The listing builds one solid part. Answer for the finished solid, in the listing's coordinates (mm). Face numbers are marked on the shaded views. A direction names the side the tool comes from. Give positions to 0.01 mm unless a question says otherwise; leave off trailing zeros. Write each loop counter-clockwise with the first axis right and the second up, starting at its lowest first coordinate (ties: lowest second). Pieces come first, ordered by that corner, then holes. Notation, with made-up numbers: (-5.75, 79.25) - (40.25, 79.25) arc R18 ccw to (40.25, 109.25) - close; hole circle Ø9 at (-23.75, 58). An arc over 180 degrees is marked (long way). Use a Markdown table: item, result. Add a question column.
from build123d import *

# Parameters (mm, degrees)
SKETCH1_R           = 1.75
SKETCH1_R_2         = 5.75
BOSS_EXTRUDE3_DEPTH = 10
FILLET1_R           = 8
SKETCH6_R           = 3.75
CUT_EXTRUDE2_DEPTH  = 3
FILLET2_R           = 8
FILLET3_R           = 3
SKETCH8_R           = 1.85
CUT_EXTRUDE3_DEPTH  = 69.282336686
SKETCH9_R           = 3.75
CUT_EXTRUDE4_DEPTH  = 4


with BuildPart() as part:
    # Sketch1 → Boss-Extrude3 (new body)
    with BuildSketch(Plane(origin=(20, 0, 0), x_dir=(0, 0, -1), z_dir=(1, 0, 0))):
        with BuildLine():
            Line((-17.699617141, 42.082180663), (-39.499785546, 42.082180663))
            Line((-39.499785546, 42.082180663), (-39.499785546, 32.582180663))
            Line((-39.499785546, 32.582180663), (-18.499785546, 32.582180663))
            Line((-18.499785546, 32.582180663), (-18.499785546, 9))
            Line((-18.499785546, 9), (-41.626388373, 9))
            ThreePointArc((-41.626388373, 9), (-51.838324672, 8.238612788), (-46.499785546, -0.5))
            Line((-46.499785546, -0.5), (-9.499785546, -0.5))
            Line((-9.499785546, -0.5), (-9.499785546, -9.5))
            Line((-9.499785546, -9.5), (9.500214454, -9.5))
            Line((9.500214454, -9.5), (9.500214454, 31.5))
            Line((9.500214454, 31.5), (-9.499785546, 31.5))
            Line((-9.499785546, 31.5), (-9.499785546, 36.5))
            ThreePointArc((-9.499785546, 36.5), (-12.123322128, 41.459787776), (-17.699617141, 42.082180663))
        make_face()
        with Locations((-15.499785546, 36.5)):
            Circle(SKETCH1_R, mode=Mode.SUBTRACT)
        with Locations((0.000214454, 22)):
            Circle(SKETCH1_R_2, mode=Mode.SUBTRACT)
        with Locations((0.000214454, 0)):
            Circle(SKETCH1_R_2, mode=Mode.SUBTRACT)
        with Locations((-15.499785546, 5.5)):
            Circle(SKETCH1_R, mode=Mode.SUBTRACT)
        with Locations((-46.499785546, 5.5)):
            Circle(SKETCH1_R, mode=Mode.SUBTRACT)
    extrude(amount=BOSS_EXTRUDE3_DEPTH)

    # Fillet1
    fillet1_edges = [part.edges().sort_by_distance(p)[0] for p in [
        (25, -9.5, 9.499785546),
        (25, -9.5, -9.500214454),
        (25, 31.5, -9.500214454),
        (25, 9, 18.499785546),
        (25, 31.5, 9.499785546),
        (25, 32.582180663, 18.499785546),
    ]]
    fillet(fillet1_edges, radius=FILLET1_R)

    # Sketch6 → Cut-Extrude2 (cut)
    with BuildSketch(Plane(origin=(30, 0, 0), x_dir=(0, 0, -1), z_dir=(1, 0, 0))):
        with Locations((-15.499785546, 36.5)):
            Circle(SKETCH6_R)
        with Locations((-15.499785546, 5.5)):
            Circle(SKETCH6_R)
        with Locations((-46.499785546, 5.5)):
            Circle(SKETCH6_R)
    extrude(amount=-CUT_EXTRUDE2_DEPTH, mode=Mode.SUBTRACT)

    # Fillet2
    fillet2_edges = [part.edges().sort_by_distance(p)[0] for p in [
        (25, -0.5, 9.499785546),
    ]]
    fillet(fillet2_edges, radius=FILLET2_R)

    # Fillet3
    fillet3_edges = [part.edges().sort_by_distance(p)[0] for p in [
        (25, 32.582180663, 39.499785546),
        (25, 42.082180663, 39.499785546),
    ]]
    fillet(fillet3_edges, radius=FILLET3_R)

    # Sketch8 → Cut-Extrude3 (cut, through all)
    with BuildSketch(Plane(origin=(30, 0, 0), x_dir=(0, 0, -1), z_dir=(1, 0, 0))):
        with Locations((-34.499785546, 37.332180663)):
            Circle(SKETCH8_R)
        with Locations((-24.499785546, 37.332180663)):
            Circle(SKETCH8_R)
    extrude(amount=-CUT_EXTRUDE3_DEPTH, mode=Mode.SUBTRACT)

    # Sketch9 → Cut-Extrude4 (cut)
    with BuildSketch(Plane.ZY.offset(-20)):
        with Locations((24.499785546, 37.332180663)):
            Circle(SKETCH9_R)
        with Locations((34.499785546, 37.332180663)):
            Circle(SKETCH9_R)
    extrude(amount=-CUT_EXTRUDE4_DEPTH, mode=Mode.SUBTRACT)


solid = part.part
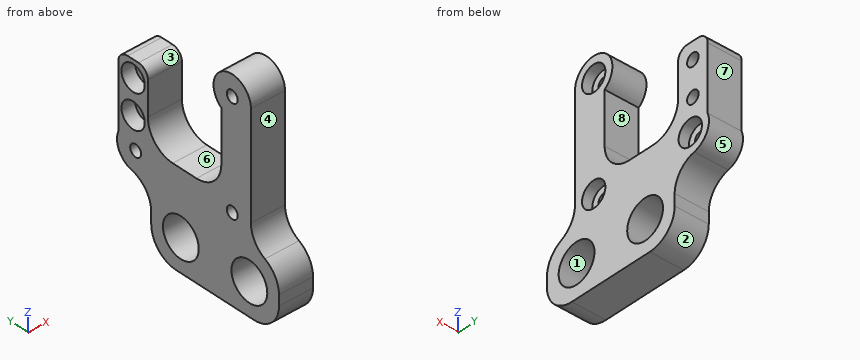
1. For a pull along Z with two mould halves and no side action, classify the marked faces 1, 2 and 3 as released by +Z, released by -Z, zero draft, split by the parting line, or undercut.
2. Which of the six approach directions +Z, -Z, +X, -X, +Y, -Y give full straight-line access (tool end or side, diameter ignored) to the marked faces 4, 5, 6, 7 and 8?
3. The part is cut by section A-A (y = 22). Give the vertices of the cut face in (x, z).
4. The part is cut by section C-C (y = 8). Give the vertices of the cut face in (x, z).
5. The part is cut by section B-B (z = 2.5). Count the separate pieces of the cut face and the enclosed holes in it, and give its area (3 significant figures).
6. Given P1, Ø5, axis at x = 25.5, z = 32, coming from the -Y side; P2, Ø1, axis at x = 25.5, z = 0.5, coming from the +Y side; P3, Ø2, axis at y = 37.33, z = 24.5, coming from the +X side; P4, Ø5, axis at x = 27.5, z = 32.5, coming from the +Y side, each flat-ended and moving along its own axis, determine where each tip first touches the part or whether it passes through.
7. Consider L1, parallel to Y at x = 21.5, z = 23; L2, parallel to Y at x = 21.75, z = 14.5; L3, parallel to Z at x = 22.75, y = 35.5. Determine where each line is inside the solid, lowest interval first. Write a range as [from, to].
Check values:
| question | item | result |
|---|---|---|
| 1 | face 1 | undercut |
| 1 | face 2 | released by -Z |
| 1 | face 3 | released by +Z |
| 2 | face 4 | +Z, +X, -X, -Y |
| 2 | face 5 | +X, -X, +Y |
| 2 | face 6 | +Z, +X, -X |
| 2 | face 7 | +Z, +X, -X, +Y |
| 2 | face 8 | +X, -X |
| 3 | outline | (20, -9.5) - (30, -9.5) - (30, -5.75) - (20, -5.75) - close; (20, 5.75) - (30, 5.75) - (30, 18.5) - (20, 18.5) - close |
| 4 | outline | (20, -9.5) - (30, -9.5) - (30, 12.7) - (27, 12.7) - (27, 18.29) - (30, 18.29) - (30, 43.7) - (27, 43.7) - (27, 49.29) - (30, 49.29) - (30, 51.95) - (20, 51.95) - close |
| 5 | separate pieces | 3 |
| 5 | enclosed holes | 0 |
| 5 | area | 203 mm2 |
| 6 | P1 | stops at y = -0.5 |
| 6 | P2 | stops at y = 31.5 |
| 6 | P3 | passes through |
| 6 | P4 | stops at y = 42.08 |
| 7 | L1 | y = [-0.5, 9.81], [31.78, 33.9], [40.77, 42.08] |
| 7 | L2 | y = [-0.62, 4.06], [6.94, 35.06], [37.94, 42.42] |
| 7 | L3 | z = [8.75, 14.06], [16.94, 21.23], [27.77, 31.23], [37.77, 39.5] |
